```python
from build123d import *

# Parameters (mm, degrees)
F0_R     = 4
F1_DEPTH = 6.35
F2_DEPTH = 355.6
F4_DEPTH = 12.7
F5_R     = 6.35
F6_DEPTH = 76.201


# Not quite as in the source:
# - a feature names something its author has since deleted; it is built from what else it names


with BuildPart() as f1:
    # F0 (on Front) → F1 (new body)
    with BuildSketch(Plane.XZ):
        with BuildLine():
            Line((-25.4, -38.65), (25.4, -38.65))
            ThreePointArc((25.4, -38.65), (29.8901280605, -36.7901280605), (31.75, -32.3))
            Line((31.75, -32.3), (31.75, 32.3))
            ThreePointArc((31.75, 32.3), (29.8901280605, 36.7901280605), (25.4, 38.65))
            Line((25.4, 38.65), (-25.4, 38.65))
            ThreePointArc((-25.4, 38.65), (-29.8901280605, 36.7901280605), (-31.75, 32.3))
            Line((-31.75, 32.3), (-31.75, -32.3))
            ThreePointArc((-31.75, -32.3), (-29.8901280605, -36.7901280605), (-25.4, -38.65))
        make_face()
        Circle(F0_R, mode=Mode.SUBTRACT)
    extrude(amount=-F1_DEPTH)

    # F0 (on Front) → F2 (join)
    with BuildSketch(Plane.XZ):
        with BuildLine():
            Line((-31.75, -45), (31.75, -45))
            ThreePointArc((31.75, -45), (36.2401280605, -43.1401280605), (38.1, -38.65))
            Line((38.1, -38.65), (38.1, 38.65))
            ThreePointArc((38.1, 38.65), (36.2401280605, 43.1401280605), (31.75, 45))
            Line((31.75, 45), (-31.75, 45))
            ThreePointArc((-31.75, 45), (-36.2401280605, 43.1401280605), (-38.1, 38.65))
            Line((-38.1, 38.65), (-38.1, -38.65))
            ThreePointArc((-38.1, -38.65), (-36.2401280605, -43.1401280605), (-31.75, -45))
        make_face()
        with BuildLine():
            ThreePointArc((31.75, -32.3), (29.8901280605, -36.7901280605), (25.4, -38.65))
            Line((25.4, -38.65), (-25.4, -38.65))
            ThreePointArc((-25.4, -38.65), (-29.8901280605, -36.7901280605), (-31.75, -32.3))
            Line((-31.75, -32.3), (-31.75, 32.3))
            ThreePointArc((-31.75, 32.3), (-29.8901280605, 36.7901280605), (-25.4, 38.65))
            Line((-25.4, 38.65), (25.4, 38.65))
            ThreePointArc((25.4, 38.65), (29.8901280605, 36.7901280605), (31.75, 32.3))
            Line((31.75, 32.3), (31.75, -32.3))
        make_face(mode=Mode.SUBTRACT)
    extrude(amount=-F2_DEPTH)

    # F0 (on Front) → F4 (join)
    with BuildSketch(Plane.XZ):
        with BuildLine():
            Line((-31.75, -45), (31.75, -45))
            ThreePointArc((31.75, -45), (36.2401280605, -43.1401280605), (38.1, -38.65))
            Line((38.1, -38.65), (38.1, 38.65))
            ThreePointArc((38.1, 38.65), (36.2401280605, 43.1401280605), (31.75, 45))
            Line((31.75, 45), (-31.75, 45))
            ThreePointArc((-31.75, 45), (-36.2401280605, 43.1401280605), (-38.1, 38.65))
            Line((-38.1, 38.65), (-38.1, -38.65))
            ThreePointArc((-38.1, -38.65), (-36.2401280605, -43.1401280605), (-31.75, -45))
        make_face()
        with BuildLine():
            ThreePointArc((31.75, -32.3), (29.8901280605, -36.7901280605), (25.4, -38.65))
            Line((25.4, -38.65), (-25.4, -38.65))
            ThreePointArc((-25.4, -38.65), (-29.8901280605, -36.7901280605), (-31.75, -32.3))
            Line((-31.75, -32.3), (-31.75, 32.3))
            ThreePointArc((-31.75, 32.3), (-29.8901280605, 36.7901280605), (-25.4, 38.65))
            Line((-25.4, 38.65), (25.4, 38.65))
            ThreePointArc((25.4, 38.65), (29.8901280605, 36.7901280605), (31.75, 32.3))
            Line((31.75, 32.3), (31.75, -32.3))
        make_face(mode=Mode.SUBTRACT)
        with BuildLine():
            Line((-25.4, -38.65), (25.4, -38.65))
            ThreePointArc((25.4, -38.65), (29.8901280605, -36.7901280605), (31.75, -32.3))
            Line((31.75, -32.3), (31.75, 32.3))
            ThreePointArc((31.75, 32.3), (29.8901280605, 36.7901280605), (25.4, 38.65))
            Line((25.4, 38.65), (-25.4, 38.65))
            ThreePointArc((-25.4, 38.65), (-29.8901280605, 36.7901280605), (-31.75, 32.3))
            Line((-31.75, 32.3), (-31.75, -32.3))
            ThreePointArc((-31.75, -32.3), (-29.8901280605, -36.7901280605), (-25.4, -38.65))
        make_face()
        Circle(F0_R, mode=Mode.SUBTRACT)
    extrude(amount=-F4_DEPTH)

    # F5 (on face) → F6 (cut, through all)
    with BuildSketch(Plane.YZ.offset(38.1)):
        with Locations((88.9, 0)):
            Circle(F5_R)
        with Locations((177.8, 0)):
            Circle(F5_R)
        with Locations((266.7, 0)):
            Circle(F5_R)
    extrude(amount=-F6_DEPTH, mode=Mode.SUBTRACT)


solid = f1.part
```
Work out the finished part from the listing and answer in its coordinate system (mm). A direction names the side the tool comes from. Coordinates: 2 decimals unless noted, no trailing zeros. Loops run counter-clockwise (first coordinate to the right, second up) from the corner with the lowest first, then second, coordinate; pieces in that order, holes last.
1) Section D-D (x = 1) is taken. Give the vertices of the cut face in (y, z), plus the area to 3 significant figures.
Results:
outline: (0, -45) - (355.6, -45) - (355.6, -38.65) - (12.7, -38.65) - (12.7, -3.87) - (0, -3.87) - close; (0, 3.87) - (12.7, 3.87) - (12.7, 38.65) - (355.6, 38.65) - (355.6, 45) - (0, 45) - close
area: 5,400 mm2
2) Section C-C (y = 41.5) is taken. Give the vertices of the cut face in (x, z), plus the area to 3 significant figures.
Results:
outline: (-38.1, -38.65) arc R6.35 ccw to (-31.75, -45) - (31.75, -45) arc R6.35 ccw to (38.1, -38.65) - (38.1, 38.65) arc R6.35 ccw to (31.75, 45) - (-31.75, 45) arc R6.35 ccw to (-38.1, 38.65) - close; hole (-31.75, -32.3) arc R6.35 ccw to (-25.4, -38.65) - (25.4, -38.65) arc R6.35 ccw to (31.75, -32.3) - (31.75, 32.3) arc R6.35 ccw to (25.4, 38.65) - (-25.4, 38.65) arc R6.35 ccw to (-31.75, 32.3) - close
area: 1,950 mm2
3) Flat-ended cylindrical pins translate along their axes: pin 1 (11.5 mm diameter, centred on y = 177.8, z = 0, fed in from +X); pin 2 (19 mm diameter, centred on x = 1, z = -3.5, fed in from +Y). Find the tip coordinate at first contact, or state that the pin passes through.
Results:
pin 1: passes through
pin 2: stops at y = 12.7
4) For a pull along Y with two mould halves and no side action, classify faces 1 (the flat face through (-9, 0, 1)), 2 (the cylindrical face through (34.969, 272.566, -2.432)), 3 (the flat face through (0, 182, -38.65)) as +Y half, -Y half, draft (parallel to the pull), parting line (faces both ways), or undercut.
Results:
face 1: -Y half
face 2: undercut
face 3: draft
5) Consider probe 1 along X at (y, z) = (227, -27.5); probe 2 along Z at (x, y) = (-17, 158.5). Determine where each line is inside the solid, lowest interval first.
Results:
probe 1: x = -38.1 to -31.75, 31.75 to 38.1
probe 2: z = -45 to -38.65, 38.65 to 45
6) Section A-A (y = 88.9) is taken. Give the vertices of the cut face in (x, z).
Results:
outline: (-38.1, -38.65) arc R6.35 ccw to (-31.75, -45) - (31.75, -45) arc R6.35 ccw to (38.1, -38.65) - (38.1, -6.35) - (31.75, -6.35) - (31.75, -32.3) arc R6.35 cw to (25.4, -38.65) - (-25.4, -38.65) arc R6.35 cw to (-31.75, -32.3) - (-31.75, -6.35) - (-38.1, -6.35) - close; (-38.1, 6.35) - (-31.75, 6.35) - (-31.75, 32.3) arc R6.35 cw to (-25.4, 38.65) - (25.4, 38.65) arc R6.35 cw to (31.75, 32.3) - (31.75, 6.35) - (38.1, 6.35) - (38.1, 38.65) arc R6.35 ccw to (31.75, 45) - (-31.75, 45) arc R6.35 ccw to (-38.1, 38.65) - close
7) Section B-B (z = 12) is taken. Give the vertices of the cut face in (x, y).
Results:
outline: (-38.1, 0) - (38.1, 0) - (38.1, 355.6) - (31.75, 355.6) - (31.75, 12.7) - (-31.75, 12.7) - (-31.75, 355.6) - (-38.1, 355.6) - close
8) For faces 4 (the cylindrical face through (36.19, 175.31, -43.19)), 5 (the flat face through (31.75, 182, -7)), determine the directions among +Z, -Z, +X, -X, +Y, -Y from which every point of the face is accessible in a straight line to the end or side of a thin tool.
Results:
face 4: -Z, +X, +Y, -Y
face 5: +Y
